```python
from build123d import *

# Parameters (mm, degrees)
SKETCH1_R           = 3.175
BOSS_EXTRUDE1_DEPTH = 12.7
SKETCH1_3_W         = 10.16
SKETCH1_3_H         = 10.16
BOSS_EXTRUDE2_DEPTH = 6.35
SKETCH2_W           = 0.527405638
SKETCH2_H           = 1.155182197
BOSS_EXTRUDE3_DEPTH = 3.048


with BuildPart() as part:
    # Sketch1 → Boss-Extrude1 (new body)
    with BuildSketch(Plane(origin=(0, 0, 0), x_dir=(1, 0, 0), z_dir=(0, 1, 0))):
        Circle(SKETCH1_R)
    extrude(amount=BOSS_EXTRUDE1_DEPTH)

    # Sketch1<3> → Boss-Extrude2 (add)
    with BuildSketch(Plane(origin=(0, 0, 0), x_dir=(1, 0, 0), z_dir=(0, 1, 0))):
        Rectangle(SKETCH1_3_W, SKETCH1_3_H)
    extrude(amount=-BOSS_EXTRUDE2_DEPTH)

    # Sketch2 → Boss-Extrude3 (add)
    with BuildSketch(Plane(origin=(5.08, 0, 0), x_dir=(0, 0, -1), z_dir=(1, 0, 0))):
        with Locations((-4.816297181, -0.577591099)):
            Rectangle(SKETCH2_W, SKETCH2_H)
        with Locations((4.816297181, -0.577591099)):
            Rectangle(SKETCH2_W, SKETCH2_H)
        with Locations((4.816297181, -5.772408902)):
            Rectangle(SKETCH2_W, SKETCH2_H)
        with Locations((-4.816297181, -5.772408902)):
            Rectangle(SKETCH2_W, SKETCH2_H)
    extrude(amount=BOSS_EXTRUDE3_DEPTH)


solid = part.part
```
Work out the finished part from the listing and answer in its coordinate system (mm). A direction names the side the tool comes from. Give positions to 0.01 mm unless a question says otherwise; leave off trailing zeros. Order: outer loops, then holes, each group sorted by start corner. A loop starts at its lowest first (then second) coordinate and runs counter-clockwise, first axis right, second up. Notation, with made-up numbers: (19, 78.25) -> (40, 78.25) arc R17 cw to (40, 90.25) -> close; hole circle Ø8 at (56, 74). An arc over 180 degrees is marked (long way). Answer as CSV lines item,"result". Start each with the question number.
(1) For a pull along Z with two mould halves and no side action, classify faces 4 (the flat face through (5.08, -3, 0)), 5 (the flat face through (1, -3, 5.08)), 6 (the flat face through (0, 12.7, 0)), 7 (the flat face through (7, -6, 4.553)) as released by +Z, released by -Z, zero draft, split by the parting line, or undercut.
(2) Which of the six approach directions +Z, -Z, +X, -X, +Y, -Y give full straight-line access (tool end or side, diameter ignored) to faces 1 (the flat face through (-5.08, -3, 0)), 2 (the flat face through (0, 0, 3.5)), 3 (the flat face through (7, -1, -4.553))?
(3) Consider line 1 along X through (y, z) = (-5.5, -3.25); line 2 along Y through (x, z) = (4, 2.75); line 3 along X through (y, z) = (9, -1). Determine where each line is inside the solid, lowest interval first.
(4) Section D-D, the plane y = 8 is taken. Write down the section's boundary in (x, z) (3 decimals).
(5) Section B-B, the plane z = 0 is taken. Write down the section's boundary in (x, y) (3 decimals), plus the area to 3 significant figures.
(6) Section C-C, the plane x = 0 is taken. Write down the section's boundary in (y, z) (3 decimals).
(7) Section A-A, the plane x = 6 is taken. Write down the section's boundary in (y, z), plus the area to 3 significant figures.
(8) Each of these flat-tipped pins is pushed along its axis until it touches: pin 1 Ø1.5 at (y, z) = (10.5, 1.5) entering from -X; pin 2 Ø2 at (x, y) = (4.5, 3.5) entering from -Z; pin 3 Ø5 at (y, z) = (-3, -2.5) entering from +X. Where does it stop, or does it pass through?
Entries:
1,face 4,"undercut"
1,face 5,"released by +Z"
1,face 6,"zero draft"
1,face 7,"undercut"
2,face 1,"+Z, -Z, -X, +Y, -Y"
2,face 2,"+Y"
2,face 3,"+X, +Y, -Y"
3,line 1,"-5.08 to 5.08"
3,line 2,"-6.35 to 0"
3,line 3,"-3.01 to 3.01"
4,outline,"circle Ø6.35 at (0, 0)"
5,outline,"(-5.08, -6.35) -> (5.08, -6.35) -> (5.08, 0) -> (3.175, 0) -> (3.175, 12.7) -> (-3.175, 12.7) -> (-3.175, 0) -> (-5.08, 0) -> close"
5,area,"145 mm²"
6,outline,"(-6.35, -5.08) -> (0, -5.08) -> (0, -3.175) -> (12.7, -3.175) -> (12.7, 3.175) -> (0, 3.175) -> (0, 5.08) -> (-6.35, 5.08) -> close"
7,outline,"(-6.35, -5.08) -> (-5.19, -5.08) -> (-5.19, -4.55) -> (-6.35, -4.55) -> close; (-6.35, 4.55) -> (-5.19, 4.55) -> (-5.19, 5.08) -> (-6.35, 5.08) -> close; (-1.16, -5.08) -> (0, -5.08) -> (0, -4.55) -> (-1.16, -4.55) -> close; (-1.16, 4.55) -> (0, 4.55) -> (0, 5.08) -> (-1.16, 5.08) -> close"
7,area,"2.44 mm²"
8,pin 1,"x = -3.09"
8,pin 2,"through"
8,pin 3,"x = 5.08"
